from build123d import *

# Parameters (mm, degrees)
SKETCH1_W                       = 15
SKETCH1_H                       = 5
BOSS_EXTRUDE1_DEPTH             = 75.2
TAP_DRILL_FOR_M3X0_5_TAP1_D     = 2.5
TAP_DRILL_FOR_M3X0_5_TAP1_DEPTH = 3
TAP_DRILL_FOR_M3X0_5_TAP1_TIP   = 0.751075774
TAP_DRILL_FOR_M3X0_5_TAP2_D     = 2.5
TAP_DRILL_FOR_M3X0_5_TAP2_DEPTH = 3
TAP_DRILL_FOR_M3X0_5_TAP2_TIP   = 0.751075774
CUT_EXTRUDE1_REACH              = 78.844
SKETCH6_R                       = 1.5
SKETCH6_R_2                     = 1
SKETCH6_W                       = 28.6
SKETCH6_H                       = 7
SKETCH6_W_2                     = 15
FILLET1_R                       = 1.5
CHAMFER1_SIZE                   = 1.5
TAP_DRILL_FOR_M3X0_5_TAP3_D     = 2.5


with BuildPart() as part:
    # Sketch1 → Boss-Extrude1 (new body)
    with BuildSketch(Plane(origin=(0, 0, 0), x_dir=(0, 0, -1), z_dir=(1, 0, 0))):
        with Locations((7.5, 2.5)):
            Rectangle(SKETCH1_W, SKETCH1_H)
    extrude(amount=BOSS_EXTRUDE1_DEPTH)

    # Tap Drill for M3x0.5 Tap1
    with Locations(Plane(origin=(75.2, 0, 0), x_dir=(0, 0, -1), z_dir=(1, 0, 0))):
        with Locations((2.5, 2.5), (12.5, 2.5)):
            Hole(TAP_DRILL_FOR_M3X0_5_TAP1_D / 2, depth=TAP_DRILL_FOR_M3X0_5_TAP1_DEPTH)
            with Locations((0, 0, -(TAP_DRILL_FOR_M3X0_5_TAP1_DEPTH + TAP_DRILL_FOR_M3X0_5_TAP1_TIP / 2))):  # 118° drill point
                Cone(0, TAP_DRILL_FOR_M3X0_5_TAP1_D / 2, TAP_DRILL_FOR_M3X0_5_TAP1_TIP, mode=Mode.SUBTRACT)

    # Tap Drill for M3x0.5 Tap2
    with Locations(Plane.ZY):
        with Locations((-2.5, 2.5), (-12.5, 2.5)):
            Hole(TAP_DRILL_FOR_M3X0_5_TAP2_D / 2, depth=TAP_DRILL_FOR_M3X0_5_TAP2_DEPTH)
            with Locations((0, 0, -(TAP_DRILL_FOR_M3X0_5_TAP2_DEPTH + TAP_DRILL_FOR_M3X0_5_TAP2_TIP / 2))):  # 118° drill point
                Cone(0, TAP_DRILL_FOR_M3X0_5_TAP2_D / 2, TAP_DRILL_FOR_M3X0_5_TAP2_TIP, mode=Mode.SUBTRACT)

    # Sketch6 → Cut-Extrude1 (cut, up to next)
    with BuildSketch(Plane(origin=(0, 5, 0), x_dir=(1, 0, 0), z_dir=(0, 1, 0)), mode=Mode.PRIVATE) as cut_extrude1_sk1:
        with Locations(Location((23.5, 3.5, 0), (0, 0, 270))):
            Circle(SKETCH6_R)
    cut_extrude1_tool1 = extrude(cut_extrude1_sk1.sketch, amount=-CUT_EXTRUDE1_REACH, mode=Mode.PRIVATE) & part.part
    # Sketch6 → Cut-Extrude1 (cut, up to next)
    with BuildSketch(Plane(origin=(0, 5, 0), x_dir=(1, 0, 0), z_dir=(0, 1, 0)), mode=Mode.PRIVATE) as cut_extrude1_sk2:
        with Locations(Location((51.7, 3.5, 0), (0, 0, 270))):
            Circle(SKETCH6_R)
    cut_extrude1_tool2 = extrude(cut_extrude1_sk2.sketch, amount=-CUT_EXTRUDE1_REACH, mode=Mode.PRIVATE) & part.part
    # Sketch6 → Cut-Extrude1 (cut, up to next)
    with BuildSketch(Plane(origin=(0, 5, 0), x_dir=(1, 0, 0), z_dir=(0, 1, 0)), mode=Mode.PRIVATE) as cut_extrude1_sk3:
        with Locations(Location((12.5, 12, 0), (0, 0, 270))):
            Circle(SKETCH6_R)
    cut_extrude1_tool3 = extrude(cut_extrude1_sk3.sketch, amount=-CUT_EXTRUDE1_REACH, mode=Mode.PRIVATE) & part.part
    # Sketch6 → Cut-Extrude1 (cut, up to next)
    with BuildSketch(Plane(origin=(0, 5, 0), x_dir=(1, 0, 0), z_dir=(0, 1, 0)), mode=Mode.PRIVATE) as cut_extrude1_sk4:
        with Locations(Location((16.5, 12, 0), (0, 0, 270))):
            Circle(SKETCH6_R_2)
    cut_extrude1_tool4 = extrude(cut_extrude1_sk4.sketch, amount=-CUT_EXTRUDE1_REACH, mode=Mode.PRIVATE) & part.part
    # Sketch6 → Cut-Extrude1 (cut, up to next)
    with BuildSketch(Plane(origin=(0, 5, 0), x_dir=(1, 0, 0), z_dir=(0, 1, 0)), mode=Mode.PRIVATE) as cut_extrude1_sk5:
        with Locations(Location((12.5, 4, 0), (0, 0, 270))):
            Circle(SKETCH6_R_2)
    cut_extrude1_tool5 = extrude(cut_extrude1_sk5.sketch, amount=-CUT_EXTRUDE1_REACH, mode=Mode.PRIVATE) & part.part
    # Sketch6 → Cut-Extrude1 (cut, up to next)
    with BuildSketch(Plane(origin=(0, 5, 0), x_dir=(1, 0, 0), z_dir=(0, 1, 0)), mode=Mode.PRIVATE) as cut_extrude1_sk6:
        with Locations(Location((16.5, 4, 0), (0, 0, 270))):
            Circle(SKETCH6_R)
    cut_extrude1_tool6 = extrude(cut_extrude1_sk6.sketch, amount=-CUT_EXTRUDE1_REACH, mode=Mode.PRIVATE) & part.part
    # Sketch6 → Cut-Extrude1 (cut, up to next)
    with BuildSketch(Plane(origin=(0, 5, 0), x_dir=(1, 0, 0), z_dir=(0, 1, 0)), mode=Mode.PRIVATE) as cut_extrude1_sk7:
        with Locations((55.9, 9.5)):
            Rectangle(SKETCH6_W, SKETCH6_H)
    cut_extrude1_tool7 = extrude(cut_extrude1_sk7.sketch, amount=-CUT_EXTRUDE1_REACH, mode=Mode.PRIVATE) & part.part
    # Sketch6 → Cut-Extrude1 (cut, up to next)
    with BuildSketch(Plane(origin=(0, 5, 0), x_dir=(1, 0, 0), z_dir=(0, 1, 0)), mode=Mode.PRIVATE) as cut_extrude1_sk8:
        with Locations((26.1, 9.5)):
            Rectangle(SKETCH6_W_2, SKETCH6_H)
    cut_extrude1_tool8 = extrude(cut_extrude1_sk8.sketch, amount=-CUT_EXTRUDE1_REACH, mode=Mode.PRIVATE) & part.part
    add(cut_extrude1_tool1.solids().sort_by_distance((23.5, 5, -3.5))[0], mode=Mode.SUBTRACT)
    add(cut_extrude1_tool2.solids().sort_by_distance((51.7, 5, -3.5))[0], mode=Mode.SUBTRACT)
    add(cut_extrude1_tool3.solids().sort_by_distance((12.5, 5, -12))[0], mode=Mode.SUBTRACT)
    add(cut_extrude1_tool4.solids().sort_by_distance((16.5, 5, -12))[0], mode=Mode.SUBTRACT)
    add(cut_extrude1_tool5.solids().sort_by_distance((12.5, 5, -4))[0], mode=Mode.SUBTRACT)
    add(cut_extrude1_tool6.solids().sort_by_distance((16.5, 5, -4))[0], mode=Mode.SUBTRACT)
    add(cut_extrude1_tool7.solids().sort_by_distance((55.9, 5, -9.5))[0], mode=Mode.SUBTRACT)
    add(cut_extrude1_tool8.solids().sort_by_distance((26.1, 5, -9.5))[0], mode=Mode.SUBTRACT)

    # Fillet1
    fillet1_edges = [part.edges().sort_by_distance(p)[0] for p in [
        (70.2, 2.5, -13),
        (70.2, 2.5, -6),
        (41.6, 2.5, -6),
        (41.6, 2.5, -13),
        (18.6, 2.5, -6),
        (18.6, 2.5, -13),
        (33.6, 2.5, -13),
        (33.6, 2.5, -6),
    ]]
    fillet(fillet1_edges, radius=FILLET1_R)

    # Chamfer1
    chamfer1_edges = [part.edges().sort_by_distance(p)[0] for p in [
        (12.5, 0, -13.5),
        (16.5, 0, -5.5),
    ]]
    chamfer(chamfer1_edges, length=CHAMFER1_SIZE - 0.0001)  # a hair under: the kernel refuses the full size

    # Tap Drill for M3x0.5 Tap3 (through all)
    with Locations(Plane(origin=(0, 5, 0), x_dir=(1, 0, 0), z_dir=(0, 1, 0))):
        with Locations((37.6, 10), (37.6, 6)):
            Hole(TAP_DRILL_FOR_M3X0_5_TAP3_D / 2)


solid = part.part
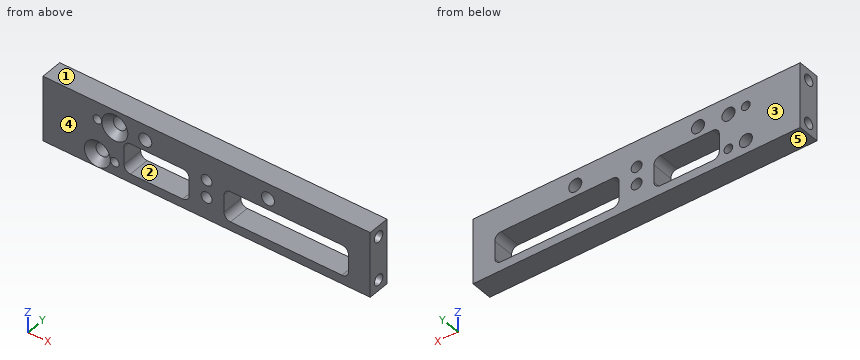
Part model, mm, in its own coordinate system. Face numbers are marked on the shaded views. A direction names the side the tool comes from. Give positions to 0.01 mm unless a question says otherwise; leave off trailing zeros. Order: outer loops, then holes, each group sorted by start corner. A loop starts at its lowest first (then second) coordinate and runs counter-clockwise, first axis right, second up. Notation, with made-up numbers: (76.25, 37.5) - (124.25, 37.5) arc R31 cw to (124.25, 76.5) - close; hole circle Ø5 at (57, -17.5). An arc over 180 degrees is marked (long way). Use a Markdown table: item, result.
1) Probe L1, parallel to X at y = 1.15, z = -10; L2, parallel to Z at x = 74.3, y = 2.5; L3, parallel to X at y = 2.9, z = -12. List the from-to ranges inside material, lowest first. Write a range as from..to.
Checked values:
| item | result |
|---|---|
| L1 | 0..18.6, 33.6..36.35, 38.85..41.6, 70.2..75.2 |
| L2 | -15..-13.75, -11.25..-3.75, -1.25..0 |
| L3 | 3.37..11, 14..15.5, 17.5..18.69, 33.51..41.69, 70.11..71.83 |
2) Saw through at C-C on x = 23.5. List the corners of the cut face in (y, z), plus the area to 3 significant figures.
Checked values:
| item | result |
|---|---|
| outline | (0, -15) - (5, -15) - (5, -13) - (0, -13) - close; (0, -6) - (5, -6) - (5, -5) - (0, -5) - close; (0, -2) - (5, -2) - (5, 0) - (0, 0) - close |
| area | 25.0 mm² |
3) Flat gauge pins, fed straight in: P1, Ø2.5, axis at x = 23.5, z = -3.5, coming from the -Y side; P2, Ø4, axis at x = 12.5, z = -12, coming from the -Y side; P3, Ø2, axis at y = 2.5, z = -12.5, coming from the -X side; P4, Ø1.5, axis at y = 2.5, z = -2.5, coming from the -X side. Where does each tip first touch, or does it go through?
Checked values:
| item | result |
|---|---|
| P1 | through |
| P2 | y = 1 |
| P3 | x = 3.15 |
| P4 | x = 3.3 |
4) Two-plate mould, pull along Y, no slides. Class the marked faces 3, 4 and 5: +Y half, -Y half, draft (parallel to the pull), parting line (faces both ways), or undercut.
Checked values:
| item | result |
|---|---|
| face 3 | +Y half |
| face 4 | -Y half |
| face 5 | draft |
5) 3-axis set-ups, long thin cutter, end or side, ignore diameter. For the marked faces 1 and 2: which of +Z, -Z, +X, -X, +Y, -Y reach the whole face in a straight line?
Checked values:
| item | result |
|---|---|
| face 1 | +Z, +X, -X, +Y, -Y |
| face 2 | +Y, -Y |
6) Saw through at A-A on x = 37.6. List the corners of the cut face in (y, z).
Checked values:
| item | result |
|---|---|
| outline | (0, -15) - (5, -15) - (5, -11.25) - (0, -11.25) - close; (0, -8.75) - (5, -8.75) - (5, -7.25) - (0, -7.25) - close; (0, -4.75) - (5, -4.75) - (5, 0) - (0, 0) - close |
7) Saw through at B-B on x = 61.5. List the corners of the cut face in (y, z), plus the area to 3 significant figures.
Checked values:
| item | result |
|---|---|
| outline | (0, -15) - (5, -15) - (5, -13) - (0, -13) - close; (0, -6) - (5, -6) - (5, 0) - (0, 0) - close |
| area | 40.0 mm² |
